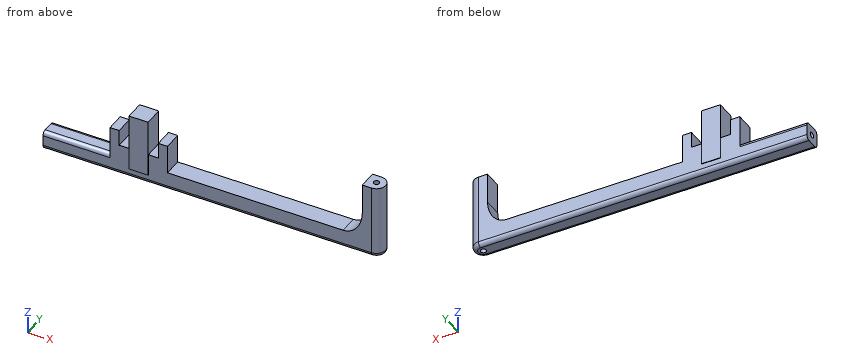
from build123d import *

# Parameters (mm, degrees)
SKETCH_1_W           = 2.4
SKETCH_1_H           = 2.4
EXTRUDE_1_DEPTH      = 7.2
EXTRUDE_2_DEPTH      = 28
EXTRUDE_2_DEPTH_BACK = 12
SKETCH_4_W           = 2.3
SKETCH_4_H           = 2.3
EXTRUDE_3_DEPTH      = 7
EXTRUDE_3_DEPTH_BACK = 2.3
SKETCH_5_R           = 0.35
SKETCH_6_R           = 0.35
CUT_EXTRUDE_1_DEPTH  = 10
FILLET_1_SIZE        = 2.4
FILLET_1_SIZE_2      = 3.2
FILLET_2_R           = 0.5
EXTRUDE_START        = -1.5
SKETCH_7_W           = 1.15
SKETCH_7_H           = 0.5
SKETCH_7_H_2         = 1.3
SKETCH_7_H_3         = 2.3
EXTRUDE_4_DEPTH      = 5.1
SKETCH_8_W           = 7.2
SKETCH_8_H           = 2.3
EXTRUDE_5_DEPTH      = 3.1


with BuildPart() as part:
    # 草图1 → 凸台-拉伸1 (new body)
    with BuildSketch(Plane.XY):
        Rectangle(SKETCH_1_W, SKETCH_1_H)
    extrude(amount=EXTRUDE_1_DEPTH)

    # 草图4 → 凸台-拉伸2 (add, two sides: drawn at the far end of the back side and taken through both)
    with BuildSketch(Plane(origin=(0, 0, 0), x_dir=(0, 0, -1), z_dir=(1, 0, 0)).offset(-EXTRUDE_2_DEPTH_BACK)):
        Rectangle(SKETCH_4_W, SKETCH_4_H)
    extrude(amount=EXTRUDE_2_DEPTH + EXTRUDE_2_DEPTH_BACK)

    # 草图5 → 凸台-拉伸3 (add, two sides: drawn at the far end of the back side and taken through both)
    with BuildSketch(Plane.XY.offset(1.15).offset(-EXTRUDE_3_DEPTH_BACK)):
        with BuildLine():
            Line((28, 0), (28, 1.15))
            Line((28, 1.15), (29.15, 1.15))
            ThreePointArc((29.15, 1.15), (30.3, 0), (29.15, -1.15))
            Line((29.15, -1.15), (28, -1.15))
            Line((28, -1.15), (28, 0))
        make_face()
        with Locations(Location((29.15, 0, 0), (0, 0, 180))):
            Circle(SKETCH_5_R, mode=Mode.SUBTRACT)
    extrude(amount=EXTRUDE_3_DEPTH + EXTRUDE_3_DEPTH_BACK)

    # 草图6 → 切除-拉伸1 (cut)
    with BuildSketch(Plane.ZY.offset(12)):
        Circle(SKETCH_6_R)
    extrude(amount=-CUT_EXTRUDE_1_DEPTH, mode=Mode.SUBTRACT)

    # 圆角1
    # an asymmetric fillet: 3.2, 2.4 mm, written as the material it adds along each edge
    with BuildSketch(Plane(origin=(28, 1.15, 1.15), x_dir=(-1, 0, 0), z_dir=(0, -1, 0))) as fillet_1_piece_1:
        with BuildLine():
            Bezier((FILLET_1_SIZE, 0), (0, 0), (0, -FILLET_1_SIZE_2), weights=[1, 0.707106781, 1])
            Line((0, -FILLET_1_SIZE_2), (0, 0))
            Line((0, 0), (FILLET_1_SIZE, 0))
        make_face()
    extrude(amount=2.3)

    # 圆角2
    fillet_2_edges = [part.edges().sort_by_distance(p)[0] for p in [
        (-6.6, -1.15, 1.15),
        (8.575, -1.15, -1.15),
        (-6.6, 1.15, 1.15),
        (8.575, 1.15, -1.15),
        (30.3, 0, -1.15),
    ]]
    fillet(fillet_2_edges, radius=FILLET_2_R)

    # 草图7 → 凸台-拉伸4 (add)
    with BuildSketch(Plane.XY.offset(1.15).offset(EXTRUDE_START)):
        with Locations((-3.025, 0.9)):
            Rectangle(SKETCH_7_W, SKETCH_7_H)
        with Locations((-3.025, 0)):
            Rectangle(SKETCH_7_W, SKETCH_7_H_2)
        with Locations((-3.025, -0.9)):
            Rectangle(SKETCH_7_W, SKETCH_7_H)
        with Locations((3.025, 0)):
            Rectangle(SKETCH_7_W, SKETCH_7_H_3)
    extrude(amount=EXTRUDE_4_DEPTH)

    # 草图8 → 凸台-拉伸5 (add)
    with BuildSketch(Plane.XY.offset(1.15).offset(EXTRUDE_START)):
        Rectangle(SKETCH_8_W, SKETCH_8_H)
    extrude(amount=EXTRUDE_5_DEPTH)


solid = part.part
The listing builds one solid part. Answer for the finished solid, in the listing's coordinates (mm). Give positions to 0.01 mm unless a question says otherwise; leave off trailing zeros. Loops run counter-clockwise (first coordinate to the right, second up) from the corner with the lowest first, then second, coordinate; pieces in that order, holes last.
Item 1: A cutting plane is placed at A-A (x = 17). Give the vertices of the cut face in (y, z).
Derived:
outline: (-1.15, -0.65) arc R0.5 ccw to (-0.65, -1.15) - (0.65, -1.15) arc R0.5 ccw to (1.15, -0.65) - (1.15, 1.15) - (-1.15, 1.15) - close
Item 2: Find the intervals of material crossed by line 1 along Y through (x, z) = (-7.25, 0); line 2 along X through (y, z) = (0.3, 5.75), in increasing order.
Derived:
line 1: y = -1.15 to -0.35, 0.35 to 1.15
line 2: x = -1.2 to 1.2, 28 to 28.97, 29.33 to 30.26
Item 3: Each of these flat-tipped pins is pushed along its axis until it touches: pin 1 Ø0.9 at (x, y) = (3, -0.5) entering from +Z; pin 2 Ø1 at (y, z) = (1, 7) entering from +X; pin 3 Ø1.4 at (x, y) = (-9.5, 0) entering from +Z. Where does it stop, or does it pass through?
Derived:
pin 1: stops at z = 4.75
pin 2: stops at x = 30.19
pin 3: stops at z = 1.15
